```python
from build123d import *

# Parameters (mm, degrees)
F0_R     = 34.925
F0_R_2   = 28.575
F1_DEPTH = 22.352
F2_R     = 7.112
F3_DEPTH = 15.748
F6_DEPTH = 14.224
F7_R     = 28.575
F8_DEPTH = 15.749


with BuildPart() as f1:
    # F0 (on Right) → F1 (new body)
    with BuildSketch(Plane.YZ):
        Circle(F0_R)
        Circle(F0_R_2, mode=Mode.SUBTRACT)
    extrude(amount=F1_DEPTH)

    # F2 (on Right) → F3 (join)
    with BuildSketch(Plane.YZ):
        with BuildLine():
            ThreePointArc((36.979548, -21.413873), (42.7322, 0), (36.979548, 21.413873))
            Line((36.979548, 21.413873), (13.627988, 61.739606))
            ThreePointArc((13.627988, 61.739606), (0, 69.596), (-13.627988, 61.739606))
            Line((-13.627988, 61.739606), (-36.979548, 21.413873))
            ThreePointArc((-36.979548, 21.413873), (-42.7322, 0), (-36.979548, -21.413873))
            Line((-36.979548, -21.413873), (-13.627988, -61.739606))
            ThreePointArc((-13.627988, -61.739606), (0, -69.596), (13.627988, -61.739606))
            Line((13.627988, -61.739606), (36.979548, -21.413873))
        make_face()
        with Locations((0, -53.848)):
            Circle(F2_R, mode=Mode.SUBTRACT)
        with Locations((0, 53.848)):
            Circle(F2_R, mode=Mode.SUBTRACT)
    extrude(amount=-F3_DEPTH)

    # F5 (on offset) → F6 (cut)
    with BuildSketch(Plane.XZ.offset(42.926)):
        with BuildLine():
            Line((-12.7, 9.54586), (-12.7, -9.75814))
            ThreePointArc((-12.7, -9.75814), (-7.874, -14.58414), (-3.048, -9.75814))
            Line((-3.048, -9.75814), (-3.048, 9.54586))
            ThreePointArc((-3.048, 9.54586), (-7.874, 14.37186), (-12.7, 9.54586))
        make_face()
    extrude(amount=-F6_DEPTH, mode=Mode.SUBTRACT)

    # F7 (on face) → F8 (cut, through all)
    with BuildSketch(Plane.YZ):
        Circle(F7_R)
    extrude(amount=-F8_DEPTH, mode=Mode.SUBTRACT)


solid = f1.part
```
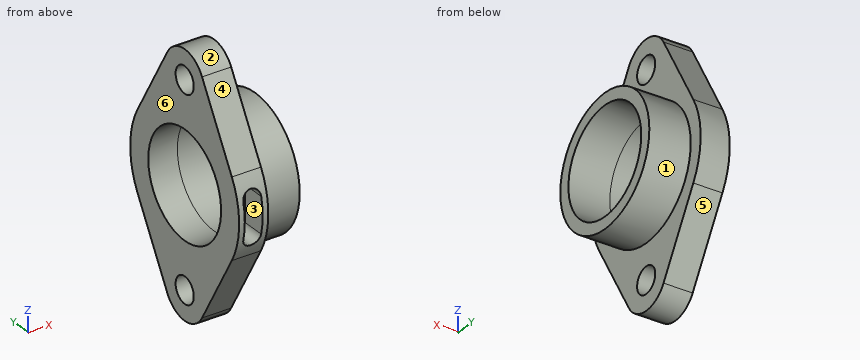
Geometry: final body of the model. Coordinates: model frame, mm. Face numbers are marked on the shaded views. A direction names the side the tool comes from. Give positions to 0.01 mm unless a question says otherwise; leave off trailing zeros. Order: outer loops, then holes, each group sorted by start corner. A loop starts at its lowest first (then second) coordinate and runs counter-clockwise, first axis right, second up. Notation, with made-up numbers: (-21.5, 27.25) -> (5.5, 27.25) arc R20 cw to (5.5, 31.25) -> close; hole circle Ø7 at (65.5, -25). An arc over 180 degrees is marked (long way). Write each question's results on one line, items separated by ' | '. Start each with the question number.
1) Line query: line 1 (Y direction, x = -13, z = -4.5); line 2 (Z direction, x = 15, y = -8); line 3 (Y direction, x = -7.5, z = 15.5). Output: solid intervals per line, ascending. Write a range as from..to.
2) Section D-D (x = 15). Return loops of the section in (y, z) (3 decimals), then the cut area to 3 significant figures.
3) Section B-B (z = 0). Return loops of the section in (x, y) (3 decimals), then the cut area to 3 significant figures.
4) Section C-C (y = 23.5). Return loops of the section in (x, z).
5) Set-up query: the marked faces 1 and 2. Return all of +Z, -Z, +X, -X, +Y, -Y with unobstructed straight access to the full face (end or side cutting, diameter ignored); none if empty.
6) Draft query along Z for the marked faces 3, 4, 5 and 6. Return one class per face: pulls with the +Z half, pulls with the -Z half, needs draft (parallel to the pull), parting line crosses it, or undercut.
7) Section A-A (y = 0). Return loops of the section in (x, z) (3 decimals), then the cut area to 3 significant figures.
8) First-contact query: pin 1 (1.5 mm diameter, centred on x = 11, y = -15, fed in from +Z); pin 2 (4 mm diameter, centred on x = 10.5, y = -3.5, fed in from -Z); pin 3 (6 mm diameter, centred on x = -10, y = -13, fed in from -Z). Flat tips, straight axial feed; report the tip coordinate or a pass-through.
Calculated:
1) line 1: -42.49..-28.22, 28.22..42.49 | line 2: -34..-27.43, 27.43..34 | line 3: -39.82..-24.01, 24.01..39.82
2) outline: circle Ø69.85 at (0, 0); hole circle Ø57.15 at (0, 0) | area: 1,270 mm2
3) outline: (-15.748, -42.732) -> (-12.7, -42.732) -> (-12.7, -28.702) -> (-3.048, -28.702) -> (-3.048, -42.732) -> (0, -42.732) -> (0, -34.925) -> (22.352, -34.925) -> (22.352, -28.575) -> (-15.748, -28.575) -> close; (-15.748, 28.575) -> (22.352, 28.575) -> (22.352, 34.925) -> (0, 34.925) -> (0, 42.732) -> (-15.748, 42.732) -> close | area: 594 mm2
4) outline: (-15.75, -44.69) -> (0, -44.69) -> (0, -25.84) -> (22.35, -25.84) -> (22.35, -16.26) -> (-15.75, -16.26) -> close; (-15.75, 16.26) -> (22.35, 16.26) -> (22.35, 25.84) -> (0, 25.84) -> (0, 44.69) -> (-15.75, 44.69) -> close
5) face 1: +X | face 2: +Z, +X, -X
6) face 3: undercut | face 4: pulls with the +Z half | face 5: pulls with the -Z half | face 6: needs draft
7) outline: (-15.748, -69.596) -> (0, -69.596) -> (0, -60.96) -> (-15.748, -60.96) -> close; (-15.748, -46.736) -> (0, -46.736) -> (0, -34.925) -> (22.352, -34.925) -> (22.352, -28.575) -> (-15.748, -28.575) -> close; (-15.748, 28.575) -> (22.352, 28.575) -> (22.352, 34.925) -> (0, 34.925) -> (0, 46.736) -> (-15.748, 46.736) -> close; (-15.748, 60.96) -> (0, 60.96) -> (0, 69.596) -> (-15.748, 69.596) -> close | area: 1,130 mm2
8) pin 1: z = 31.89 | pin 2: z = -34.89 | pin 3: z = -66.01
